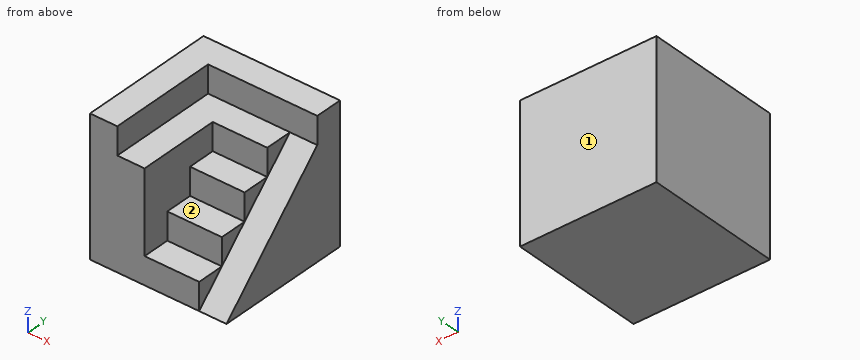
```python
from build123d import *

# Parameters (mm, degrees)
F1_DEPTH = 32
F3_DEPTH = 25
F4_DEPTH = 40
F0_W     = 8
F0_H     = 8
F5_DEPTH = 40
F6_DEPTH = 32
F0_W_2   = 16
F7_DEPTH = 24
F8_DEPTH = 16
F9_DEPTH = 8


with BuildPart() as f1:
    # F0 (on Top) → F1 (new body)
    with BuildSketch(Plane.XY):
        Polygon((20, 12), (12, 12), (12, 4), (12, -4), (12, -12), (12, -20), (20, -20), align=None)
    extrude(amount=F1_DEPTH)

    # F2 (on face) → F3 (cut)
    with BuildSketch(Plane.YZ.offset(20)):
        Polygon((-20, 0), (12, 32), (-20, 32), align=None)
    extrude(amount=-F3_DEPTH, mode=Mode.SUBTRACT)

    # F0 (on Top) → F4 (join)
    with BuildSketch(Plane.XY):
        Polygon((12, 20), (-20, 20), (-20, -20), (-12, -20), (-12, 12), (12, 12), align=None)
    extrude(amount=F4_DEPTH)

    # F0 (on Top) → F5 (join)
    with BuildSketch(Plane.XY):
        with Locations((16, 16)):
            Rectangle(F0_W, F0_H)
    extrude(amount=F5_DEPTH)

    # F0 (on Top) → F6 (join)
    with BuildSketch(Plane.XY):
        Polygon((12, 4), (12, 12), (-12, 12), (-12, -20), (-4, -20), (-4, -12), (-4, -4), (-4, 4), align=None)
    extrude(amount=F6_DEPTH)

    # F0 (on Top) → F7 (join)
    with BuildSketch(Plane.XY):
        with Locations((4, 0)):
            Rectangle(F0_W_2, F0_H)
    extrude(amount=F7_DEPTH)

    # F0 (on Top) → F8 (join)
    with BuildSketch(Plane.XY):
        with Locations((4, -8)):
            Rectangle(F0_W_2, F0_H)
    extrude(amount=F8_DEPTH)

    # F0 (on Top) → F9 (join)
    with BuildSketch(Plane.XY):
        with Locations((4, -16)):
            Rectangle(F0_W_2, F0_H)
    extrude(amount=F9_DEPTH)


solid = f1.part
```
The model under review builds one solid part; all positions refer to its coordinate system, in mm. Face numbers are marked on the shaded views. A direction names the side the tool comes from. Round coordinates to 2 decimals unless told otherwise and drop trailing zeros. Loops run counter-clockwise (first coordinate to the right, second up) from the corner with the lowest first, then second, coordinate; pieces in that order, holes last.
Item 1: Take a section at C-C (x = 4). Write out the cut boundary in (y, z).
Determined:
outline: (-20, 0) - (20, 0) - (20, 40) - (12, 40) - (12, 32) - (4, 32) - (4, 24) - (-4, 24) - (-4, 16) - (-12, 16) - (-12, 8) - (-20, 8) - close
Item 2: Clearance check with flat-ended pins moving along their axes: pin 1 Ø9 at (y, z) = (-3.5, 37.5) entering from +X; pin 2 Ø5 at (y, z) = (-2.5, 29) entering from +X; pin 3 Ø4 at (x, y) = (1.5, 1) entering from +Z. State where each tip first meets the part, or that it passes through.
Determined:
pin 1: stops at x = -12
pin 2: stops at x = -4
pin 3: stops at z = 24
Item 3: Take a section at B-B (y = 0). Write out the cut boundary in (x, z), then the cut area to 3 significant figures.
Determined:
outline: (-20, 0) - (20, 0) - (20, 20) - (12, 20) - (12, 24) - (-4, 24) - (-4, 32) - (-12, 32) - (-12, 40) - (-20, 40) - close
area: 1,120 mm2
Item 4: Take a section at D-D (z = 31). Write out the cut boundary in (x, y), then the cut area to 3 significant figures.
Determined:
outline: (-20, -20) - (-4, -20) - (-4, 4) - (12, 4) - (12, 11) - (20, 11) - (20, 20) - (-20, 20) - close
area: 968 mm2
Item 5: For the marked faces 1 and 2, list the 3-axis set-ups (+Z, -Z, +X, -X, +Y, -Y) from which the entire face can be reached by the end or side of a thin tool; tool diameter is ignored.
Determined:
face 1: +Z, -Z, +X, -X, +Y
face 2: +Z, +X, -Y
Item 6: For line 1 (Z direction, x = 8, y = 7.5); line 2 (Y direction, x = 5.5, z = 21.5); line 3 (Y direction, x = 0.5, z = 36), list the stretches that pass through material, from the lowest coordinate up.
Determined:
line 1: z = 0 to 32
line 2: y = -4 to 20
line 3: y = 12 to 20
Item 7: Take a section at A-A (z = 19). Write out the cut boundary in (x, y).
Determined:
outline: (-20, -20) - (-4, -20) - (-4, -4) - (12, -4) - (12, -1) - (20, -1) - (20, 20) - (-20, 20) - close
